Check sheet for the drawn part. Datum: minimum x, y, z corner. Units: mm. A direction names the side the tool comes from. Coordinates: 2 decimals unless noted, no trailing zeros. Loops run counter-clockwise (first coordinate to the right, second up) from the corner with the lowest first, then second, coordinate; pieces in that order, holes last. Notation, with made-up numbers: M 55,39 L 81,39 A32 cw 81,77 Z; hole C 15,-17 d11. An arc over 180 degrees is marked long. Answer in a Markdown table with one row per item. Add a question column.
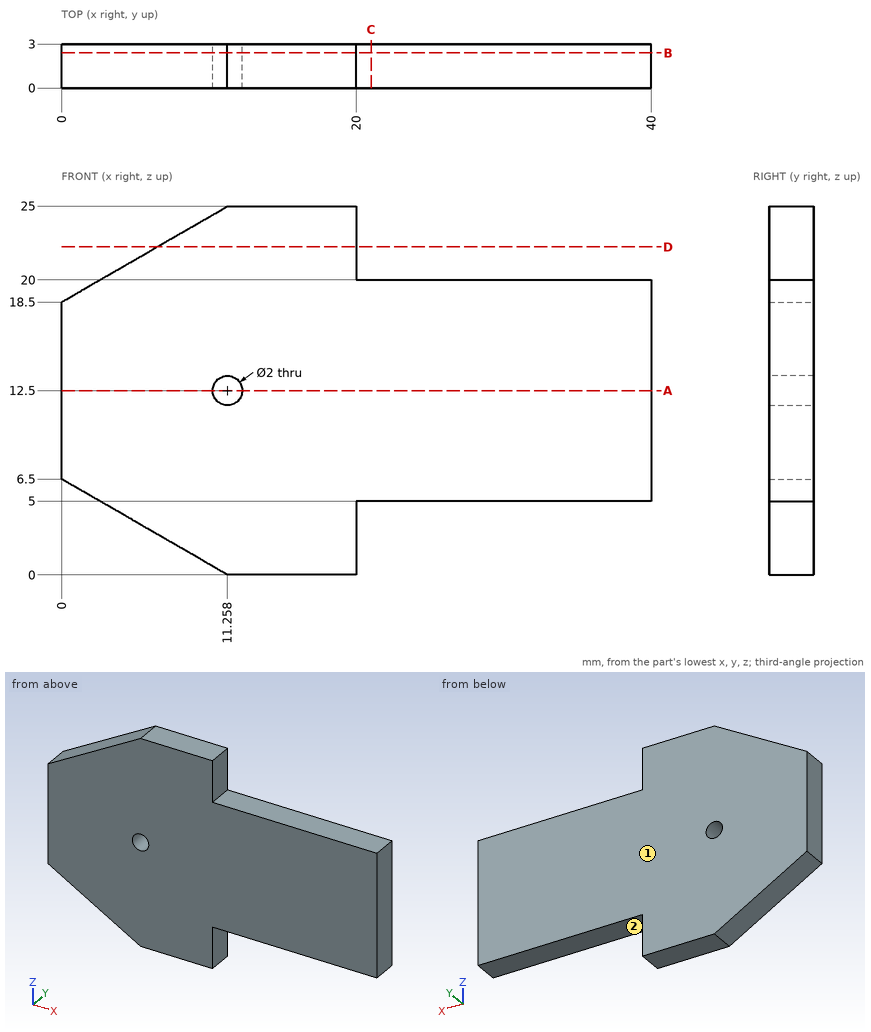
Q1. Cross-section at C-C (x = 21). Record the cut outline in (y, z).
Q2. Go/stop test with flat-tipped pins: pin 1 (1 mm diameter, centred on x = 8.5, y = 1.5, fed in from -Z); pin 2 (0.9 mm diameter, centred on x = 33.5, y = 2, fed in from -Z); pin 3 (1.5 mm diameter, centred on y = 2, z = 23, fed in from +X). Record where each tip stops, or that it passes through.
Q3. Access from +Z, -Z, +X, -X, +Y, -Y to the whole of each face (thin tool, end or side, straight path). Record for the marked faces 1 and 2.
Q4. Thickness scan on L1, parallel to X at y = 1.25, z = 12.5; L2, parallel to Z at x = 33, y = 0.65; L3, parallel to X at y = 0.2, z = 13.25 (1 decimal). Record the ranges inside material, lowest first.
Q5. Cross-section at D-D (z = 22.25). Record the cut outline in (x, y) (1 decimal), plus the area to 3 significant figures.
Q6. Cross-section at A-A (z = 12.5). Record the cut outline in (x, y), plus the area to 3 significant figures.
Q7. Cross-section at B-B (y = 2.4). Record the cut outline in (x, z).
Answer key:
| question | item | result |
|---|---|---|
| 1 | outline | M 0,5 L 3,5 L 3,20 L 0,20 Z |
| 2 | pin 1 | z = 1.3 |
| 2 | pin 2 | z = 5 |
| 2 | pin 3 | x = 20 |
| 3 | face 1 | +Z, -Z, +X, -X, +Y |
| 3 | face 2 | -Z, +X, +Y, -Y |
| 4 | L1 | 0 to 10.26, 12.26 to 40 |
| 4 | L2 | 5 to 20 |
| 4 | L3 | 0 to 10.6, 11.9 to 40 |
| 5 | outline | M 6.5,0 L 20,0 L 20,3 L 6.5,3 Z |
| 5 | area | 40.5 mm^2 |
| 6 | outline | M 0,0 L 10.26,0 L 10.26,3 L 0,3 Z; M 12.26,0 L 40,0 L 40,3 L 12.26,3 Z |
| 6 | area | 114 mm^2 |
| 7 | outline | M 0,6.5 L 11.26,0 L 20,0 L 20,5 L 40,5 L 40,20 L 20,20 L 20,25 L 11.26,25 L 0,18.5 Z; hole C 11.26,12.5 d2 |
